Could you check a few things on this drawing? It's one solid part, dimensions in mm from its lowest x, y, z. A direction names the side the tool comes from. Coordinates: 2 decimals unless noted, no trailing zeros. Write each loop counter-clockwise with the first axis right and the second up, starting at its lowest first coordinate (ties: lowest second). Pieces come first, ordered by that corner, then holes. Notation, with made-up numbers: (-26, -11.75) - (-1, -11.75) arc R8 ccw to (-1, -2.75) - close; hole circle Ø6 at (-3.5, 26). An arc over 180 degrees is marked (long way). Use one line per item in the form item = value. Start each with the question number.
(1) For pin 1 Ø4 at (x, y) = (94.5, 40.5) entering from +Z; pin 2 Ø4 at (y, z) = (42.5, 17) entering from +X; pin 3 Ø4 at (y, z) = (41.5, 18.5) entering from -X, each with a flat end and sliding along its axis, tell me the tip position at first contact or that it passes through.
(2) If we section it at A-A on x = 3.5: Please give me the cut outline in (y, z).
(3) If we section it at B-B on y = 3.9: Please give me the cut outline in (x, z), then the cut area to 3 significant figures.
(4) On a 3-axis mill with a long thin cutter (end or side, diameter ignored), from which of +Z, -Z, +X, -X, +Y, -Y can I reach the whole of each face in a straight line? I mean the marked faces 1, 2 and 3. Say none if no direction works.
(5) If we section it at C-C on z = 21: Please give me the cut outline in (x, y).
(6) If I drill on probe 1 along Y at (x, z) = (96.5, 0.3); probe 2 along X at (y, z) = (41.5, 19.25), over which ranges is the centre line in solid material (lowest first)? Write a range as from..to.
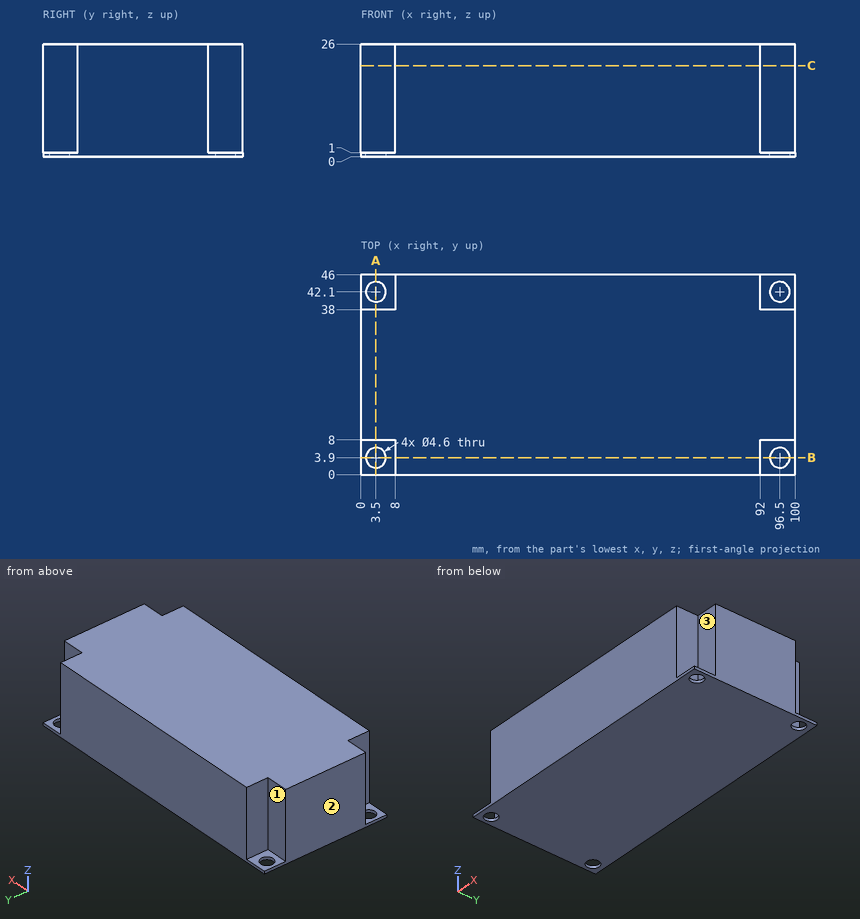
Reported:
q1.pin_1 = 1
q1.pin_2 = 92
q1.pin_3 = 8
q2.outline = (0, 0) - (1.6, 0) - (1.6, 1) - (0, 1) - close; (6.2, 0) - (39.8, 0) - (39.8, 1) - (38, 1) - (38, 26) - (8, 26) - (8, 1) - (6.2, 1) - close; (44.4, 0) - (46, 0) - (46, 1) - (44.4, 1) - close
q3.outline = (0, 0) - (1.2, 0) - (1.2, 1) - (0, 1) - close; (5.8, 0) - (94.2, 0) - (94.2, 1) - (92, 1) - (92, 26) - (8, 26) - (8, 1) - (5.8, 1) - close; (98.8, 0) - (100, 0) - (100, 1) - (98.8, 1) - close
q3.area = 2,190 mm2
q4.face_1 = +Z, -X, +Y
q4.face_2 = +Z, -Z, -X, +Y, -Y
q4.face_3 = +Z, +X, -Y
q5.outline = (0, 8) - (8, 8) - (8, 0) - (92, 0) - (92, 8) - (100, 8) - (100, 38) - (92, 38) - (92, 46) - (8, 46) - (8, 38) - (0, 38) - close
q6.probe_1 = 0..1.6, 6.2..39.8, 44.4..46
q6.probe_2 = 8..92
